Answer from the drawing. Dimensions are ordinates in mm from the lowest x, y and z of the part. Give positions to 0.01 mm unless a question says otherwise; leave off trailing zeros. Order: outer loops, then holes, each group sorted by start corner. A loop starts at its lowest first (then second) coordinate and runs counter-clockwise, first axis right, second up. Notation, with made-up numbers: (-13, 47) - (2, 47) arc R24 ccw to (2, 82) - close; hole circle Ø7 at (-15.5, 33). An arc over 180 degrees is marked (long way). Write each question's results on one line, items separated by ' | '.
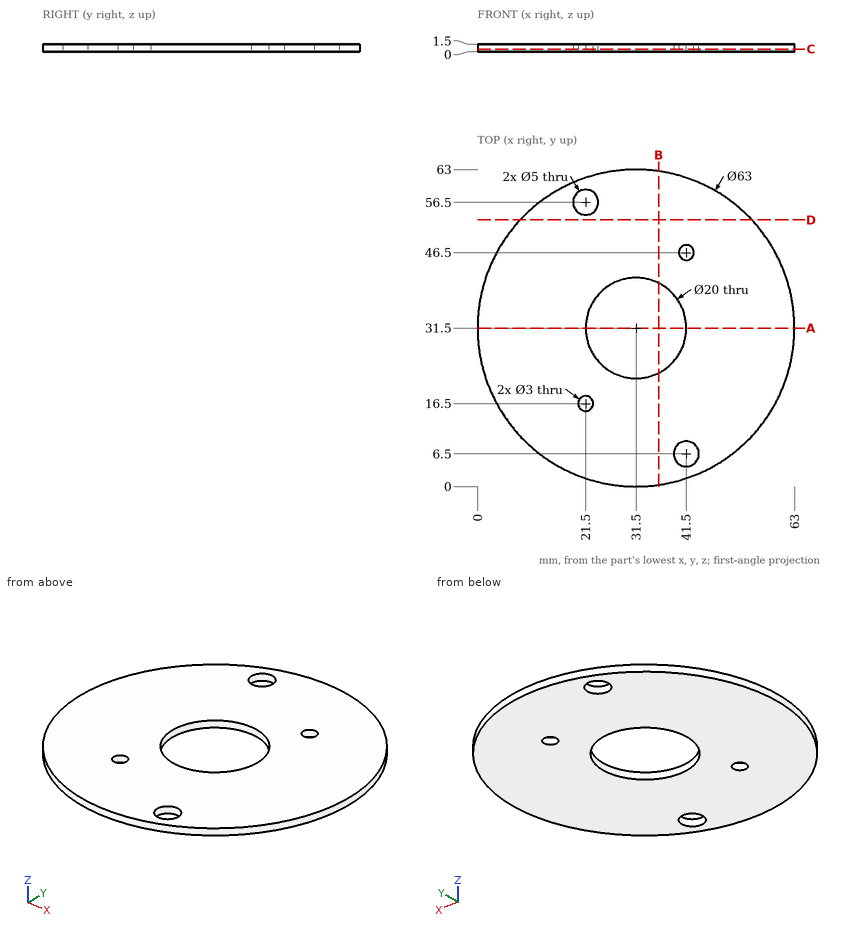
(1) This flat-tipped pin is pushed along its axis until it touches: pin 1 (1.8 mm diameter, centred on x = 21.5, y = 16.5, fed in from -Z). Where does it stop, or does it pass through?
Conclusion:
pin 1: through
(2) Section D-D (y = 53) is taken. Give the vertices of the cut face in (x, z), plus the area to 3 significant figures.
Conclusion:
outline: (8.48, 0) - (54.52, 0) - (54.52, 1.5) - (8.48, 1.5) - close | area: 69.1 mm^2
(3) Section B-B (x = 36) is taken. Give the vertices of the cut face in (y, z).
Conclusion:
outline: (0.32, 0) - (22.57, 0) - (22.57, 1.5) - (0.32, 1.5) - close; (40.43, 0) - (62.68, 0) - (62.68, 1.5) - (40.43, 1.5) - close
(4) Section C-C (z = 0.5) is taken. Give the vertices of the cut face in (x, y).
Conclusion:
outline: circle Ø63 at (31.5, 31.5); hole circle Ø5 at (21.5, 56.5); hole circle Ø3 at (21.5, 16.5); hole circle Ø20 at (31.5, 31.5); hole circle Ø5 at (41.5, 6.5); hole circle Ø3 at (41.5, 46.5)
(5) Consider probe 1 along Y at (x, z) = (31.5, 0.45); probe 2 along X at (y, z) = (26, 1); probe 3 along X at (y, z) = (38, 1.25). Determine where each line is inside the solid, lowest interval first. Write a range as [from, to].
Conclusion:
probe 1: [0, 21.5], [41.5, 63] | probe 2: [0.48, 23.15], [39.85, 62.52] | probe 3: [0.68, 23.9], [39.1, 62.32]
(6) Section A-A (y = 31.5) is taken. Give the vertices of the cut face in (x, z).
Conclusion:
outline: (0, 0) - (21.5, 0) - (21.5, 1.5) - (0, 1.5) - close; (41.5, 0) - (63, 0) - (63, 1.5) - (41.5, 1.5) - close
